Work out the finished part from the listing and answer in its coordinate system (mm). Face numbers are marked on the shaded views. A direction names the side the tool comes from. Round coordinates to 2 decimals unless told otherwise and drop trailing zeros. Order: outer loops, then holes, each group sorted by start corner. A loop starts at its lowest first (then second) coordinate and runs counter-clockwise, first axis right, second up. Notation, with made-up numbers: (35.5, 83.25) -> (47.5, 83.25) arc R24 cw to (47.5, 106.25) -> close; hole circle Ø4 at (42.5, 76.25). An arc over 180 degrees is marked (long way). Use one line per item in the form item = value.
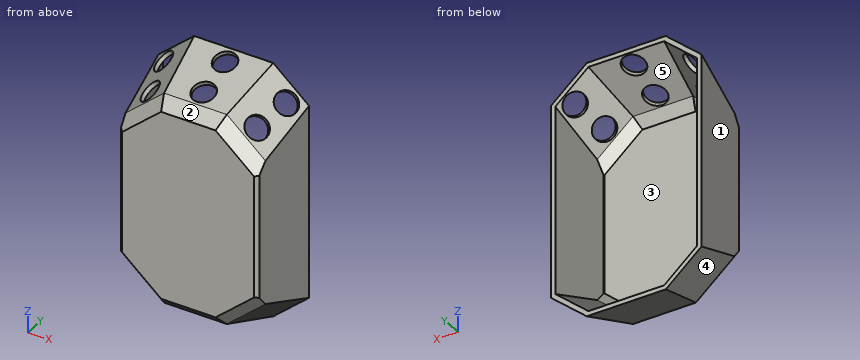
```python
from build123d import *
from OCP.BRepFilletAPI import BRepFilletAPI_MakeChamfer

# Parameters (mm, degrees)
SKETCH1_W             = 96.449496644
SKETCH1_H             = 93.866027984
BOSS_EXTRUDE1_DEPTH   = 50
DRAFT1_ANGLE          = 20
DRAFT2_ANGLE          = 5
CHAMFER1_SIZE         = 5
CHAMFER1_SIZE2        = 8.365785926
CHAMFER1_EDGE_2_SIZE  = 5
CHAMFER1_EDGE_2_SIZE2 = 8.365785926
CHAMFER1_EDGE_3_SIZE  = 5
CHAMFER1_EDGE_3_SIZE2 = 8.365785926
CHAMFER1_EDGE_4_SIZE  = 5
CHAMFER1_EDGE_4_SIZE2 = 8.365785926
CHAMFER1_EDGE_5_SIZE  = 5
CHAMFER1_EDGE_5_SIZE2 = 8.365785926
CHAMFER1_EDGE_6_SIZE  = 5
CHAMFER1_EDGE_6_SIZE2 = 8.365785926
CHAMFER2_SIZE         = 2
CHAMFER2_SIZE2        = 2.200125735
SHELL1_T              = -3
SKETCH2_R             = 8
CUT_EXTRUDE1_DEPTH    = 174.798113009
SKETCH3_R             = 8
CUT_EXTRUDE2_DEPTH    = 173.570101234


with BuildPart() as part:
    # Sketch1 → Boss-Extrude1 (new body)
    with BuildSketch(Plane(origin=(0, 0, 0), x_dir=(1, 0, 0), z_dir=(0, 1, 0))):
        Rectangle(SKETCH1_W, SKETCH1_H)
        Polygon((20.883038336, 70.399520989), (48.224748322, 46.933013992), (-48.224748322, 46.933013992), (-20.883038336, 70.399520989), align=None)
        Polygon((-48.224748322, -46.933013992), (48.224748322, -46.933013992), (20.883038336, -70.399520989), (-20.883038336, -70.399520989), align=None)
    extrude(amount=BOSS_EXTRUDE1_DEPTH)

    # Draft1
    draft1_faces = [part.faces().sort_by_distance(p)[0] for p in [
        (-34.553893329, 25, 58.66626749),
        (-34.553893329, 25, -58.66626749),
        (0, 25, -70.399520989),
        (34.553893329, 25, -58.66626749),
        (34.553893329, 25, 58.66626749),
        (0, 25, 70.399520989),
    ]]
    draft(draft1_faces, Plane(origin=(0, 0, 0), x_dir=(0, 0, -1), z_dir=(0, -1, 0)), DRAFT1_ANGLE)

    # Draft2
    draft2_faces = [part.faces().sort_by_distance(p)[0] for p in [
        (48.224748322, 26.695838409, 0),
        (-48.224748322, 26.695838409, 0),
    ]]
    draft(draft2_faces, Plane(origin=(0, 0, 0), x_dir=(0, 0, -1), z_dir=(0, -1, 0)), DRAFT2_ANGLE)

    # Chamfer1
    chamfer1_edges = [part.edges().sort_by_distance(p)[0] for p in [
        (0, 0, 70.399520989),
    ]]
    chamfer1_side = [part.faces().sort_by_distance(p)[0] for p in [
        (0, 0, 0),
    ]]
    chamfer(chamfer1_edges, length=CHAMFER1_SIZE, length2=CHAMFER1_SIZE2, reference=chamfer1_side[0])

    # Chamfer1 edge 2
    chamfer1_edge_2_edges = [part.edges().sort_by_distance(p)[0] for p in [
        (-34.553893329, 0, 58.66626749),
    ]]
    chamfer1_edge_2_side = [part.faces().sort_by_distance(p)[0] for p in [
        (0, 0, 0),
    ]]
    chamfer(chamfer1_edge_2_edges, length=CHAMFER1_EDGE_2_SIZE, length2=CHAMFER1_EDGE_2_SIZE2, reference=chamfer1_edge_2_side[0])

    # Chamfer1 edge 3
    chamfer1_edge_3_edges = [part.edges().sort_by_distance(p)[0] for p in [
        (-34.553893329, 0, -58.66626749),
    ]]
    chamfer1_edge_3_side = [part.faces().sort_by_distance(p)[0] for p in [
        (0, 0, 0),
    ]]
    chamfer(chamfer1_edge_3_edges, length=CHAMFER1_EDGE_3_SIZE, length2=CHAMFER1_EDGE_3_SIZE2, reference=chamfer1_edge_3_side[0])

    # Chamfer1 edge 4
    chamfer1_edge_4_edges = [part.edges().sort_by_distance(p)[0] for p in [
        (0, 0, -70.399520989),
    ]]
    chamfer1_edge_4_side = [part.faces().sort_by_distance(p)[0] for p in [
        (0, 0, 0),
    ]]
    chamfer(chamfer1_edge_4_edges, length=CHAMFER1_EDGE_4_SIZE, length2=CHAMFER1_EDGE_4_SIZE2, reference=chamfer1_edge_4_side[0])

    # Chamfer1 edge 5
    chamfer1_edge_5_edges = [part.edges().sort_by_distance(p)[0] for p in [
        (34.553893329, 0, -58.66626749),
    ]]
    chamfer1_edge_5_side = [part.faces().sort_by_distance(p)[0] for p in [
        (0, 0, 0),
    ]]
    chamfer(chamfer1_edge_5_edges, length=CHAMFER1_EDGE_5_SIZE, length2=CHAMFER1_EDGE_5_SIZE2, reference=chamfer1_edge_5_side[0])

    # Chamfer1 edge 6
    chamfer1_edge_6_edges = [part.edges().sort_by_distance(p)[0] for p in [
        (34.553893329, 0, 58.66626749),
    ]]
    chamfer1_edge_6_side = [part.faces().sort_by_distance(p)[0] for p in [
        (0, 0, 0),
    ]]
    chamfer(chamfer1_edge_6_edges, length=CHAMFER1_EDGE_6_SIZE, length2=CHAMFER1_EDGE_6_SIZE2, reference=chamfer1_edge_6_side[0])

    # Chamfer2: one chamfer whose edges measure the first distance from different faces: ONE call of the kernel's chamfer builder (chamfer() names one face for all edges)
    chamfer2_edges_1 = [part.edges().sort_by_distance(p)[0] for p in [
        (48.224748322, 0, 0),
    ]]
    chamfer2_side_1 = [part.faces().sort_by_distance(p)[0] for p in [
        (50.560348002, 26.696026495, 0),
    ]]
    chamfer2_edges_2 = [part.edges().sort_by_distance(p)[0] for p in [
        (-48.224748322, 0, 0),
    ]]
    chamfer2_side_2 = [part.faces().sort_by_distance(p)[0] for p in [
        (0, 0, 0),
    ]]
    chamfer2 = BRepFilletAPI_MakeChamfer(part.part.solid().wrapped)
    for e in chamfer2_edges_1:
        chamfer2.Add(CHAMFER2_SIZE, CHAMFER2_SIZE2, e.wrapped, chamfer2_side_1[0].wrapped)  # the first distance lies on this face
    for e in chamfer2_edges_2:
        chamfer2.Add(CHAMFER2_SIZE, CHAMFER2_SIZE2, e.wrapped, chamfer2_side_2[0].wrapped)  # the first distance lies on this face
    add(Compound.cast(chamfer2.Shape()), mode=Mode.REPLACE)

    # Shell1
    shell1_openings = [part.faces().sort_by_distance(p)[0] for p in [
        (0, 50, 0),
    ]]
    offset(amount=SHELL1_T, openings=shell1_openings, kind=Kind.INTERSECTION)

    # Sketch2 → Cut-Extrude1 (cut, through all)
    with BuildSketch(Plane(origin=(36.708388619, -20.5145146, 42.770324355), x_dir=(-0.7908530317789993, -0.26467423150818037, 0.5518143105262125), z_dir=(-0.6120061128174825, 0.3420201433256695, -0.7130713424570668))):
        with Locations(Location((-5.537538823, 67.111220428, 0), (0, 0, 16.359329629))):
            Circle(SKETCH2_R)
        with Locations(Location((1.503972029, 43.123366733, 0), (0, 0, 16.359329629))):
            Circle(SKETCH2_R)
    cut_extrude1 = extrude(amount=-CUT_EXTRUDE1_DEPTH, mode=Mode.SUBTRACT)

    # Sketch3 → Cut-Extrude2 (cut, through all)
    with BuildSketch(Plane(origin=(0, -21.59990948, 59.345263558), x_dir=(-1, 0, 0), z_dir=(0, 0.34202014332566943, -0.9396926207859082))):
        with Locations(Location((0, 67.108924172, 0), (0, 0, 90))):
            Circle(SKETCH3_R)
        with Locations(Location((0, 42.108924172, 0), (0, 0, 90))):
            Circle(SKETCH3_R)
    extrude(amount=-CUT_EXTRUDE2_DEPTH, mode=Mode.SUBTRACT)

    # Mirror1: Cut-Extrude1 across plane
    add(cut_extrude1.mirror(Plane(origin=(0, 0, 0), x_dir=(0, 0, 1), z_dir=(1, 0, 0))), mode=Mode.SUBTRACT)


solid = part.part
```
Item 1: The part is cut by section A-A, the plane z = 25.5. Give the vertices of the cut face in (x, y), and give its area (3 significant figures).
Findings:
outline = (-52.6, 50) -> (-48.42, 2.19) -> (-46.22, 0) -> (46.02, 0) -> (48.4, 1.99) -> (52.6, 50) -> (49.59, 50) -> (45.52, 3.49) -> (44.93, 3) -> (-44.98, 3) -> (-45.52, 3.54) -> (-49.59, 50) -> close
area = 569 mm^2
Item 2: The part is cut by section C-C, the plane y = 22. Give the number of separate pieces and of enclosed holes in the cut face, and give its area (3 significant figures).
Findings:
separate_pieces = 3
enclosed_holes = 0
area = 1,270 mm^2
Item 3: Consider line 1 along Y through (x, z) = (28, 47); line 2 along X through (y, z) = (43.5, 45); line 3 along X through (y, z) = (14, 20.5). Determine where each line is inside the solid, lowest interval first.
Findings:
line_1 = 0 to 3
line_2 = -52.03 to -49.02, 49.02 to 52.03
line_3 = -49.45 to -46.44, 46.44 to 49.45
Item 4: The part is cut by section B-B, the plane x = 11.5. Give the vertices of the cut face in (y, z), and give its area (3 significant figures).
Findings:
outline = (0, -65.4) -> (7.86, -73.26) -> (50, -88.6) -> (50, -85.41) -> (9.51, -70.67) -> (3, -64.16) -> (3, 64.16) -> (9.51, 70.67) -> (50, 85.41) -> (50, 88.6) -> (7.86, 73.26) -> (0, 65.4) -> close
area = 713 mm^2
Item 5: Determine the mould class of the marked faces 1, 2 and 3 for opening direction X: released by +X, released by -X, zero draft, split by the parting line, or undercut.
Findings:
face_1 = released by -X
face_2 = zero draft
face_3 = undercut
Item 6: Flat-ended cylindrical pins translate along their axes: P1, Ø6, axis at x = -9.5, y = 35.5, coming from the +Z side; P2, Ø10, axis at x = 21.5, y = 25, coming from the +Z side; P3, Ø10, axis at x = 32, y = 32.5, coming from the +Z side. Find the tip coordinate at first contact, or state that the pin passes through.
Findings:
P1 = 84.41
P2 = 81.32
P3 = 81.36
Item 7: For the marked faces 4 and 5, determine the directions among +Z, -Z, +X, -X, +Y, -Y from which every point of the face is accessible in a straight line to the end or side of a thin tool.
Findings:
face_4 = -Z, -X, -Y
face_5 = +Y
